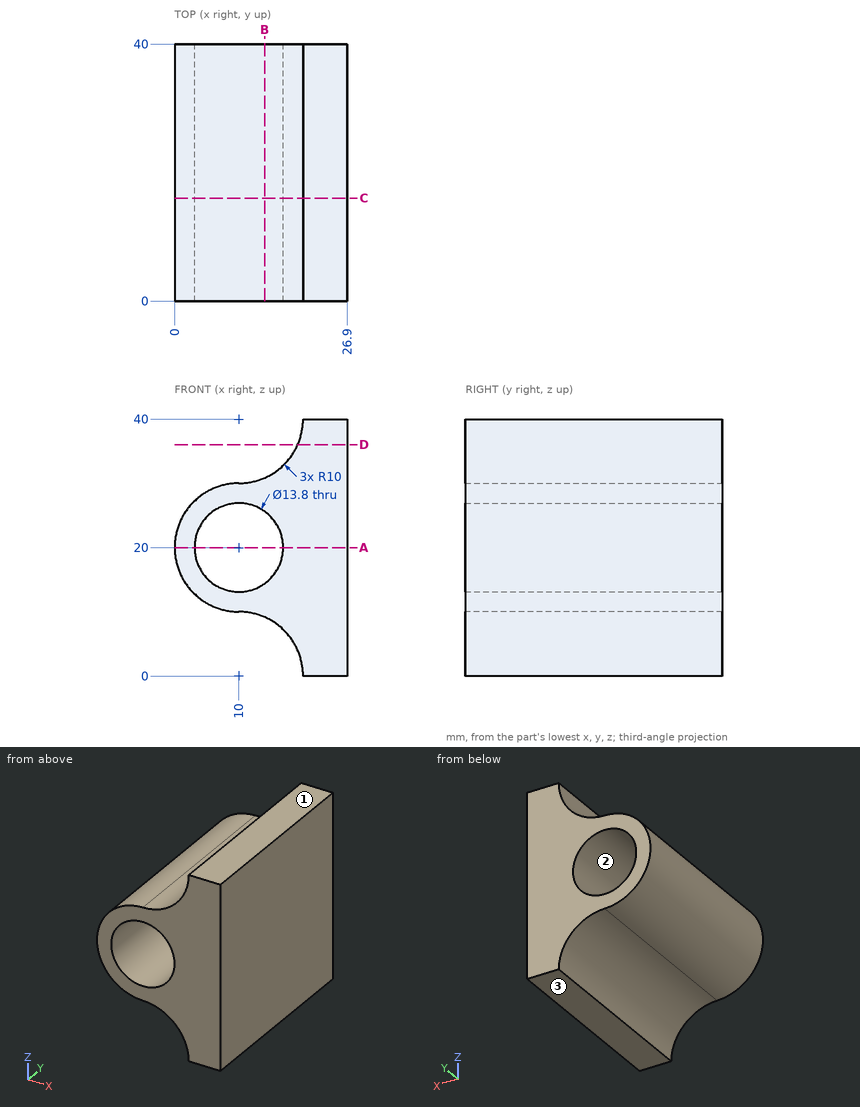
Geometry: see drawing. Coordinates: mm, zero at the bounding-box minimum. Coordinates: 2 decimals unless noted, no trailing zeros. Order: outer loops, then holes, each group sorted by start corner. A loop starts at its lowest first (then second) coordinate and runs counter-clockwise, first axis right, second up. Notation, with made-up numbers: (88, 70.5) - (145, 70.5) arc R15 ccw to (145, 77.5) - close; hole circle Ø11 at (89.5, 6). An arc over 180 degrees is marked (long way). Use one line per item in the form item = value.
1) Section C-C (y = 16). Return loops of the section in (x, z), then the cut area to 3 significant figures.
Solutions:
outline = (10, 10) arc R10 cw to (20, 0) - (26.9, 0) - (26.9, 40) - (20, 40) arc R10 cw to (10, 30) arc R10 ccw to start; hole circle Ø13.8 at (10, 20)
area = 526 mm^2
2) Section A-A (z = 20). Return loops of the section in (x, y).
Solutions:
outline = (0, 0) - (3.1, 0) - (3.1, 40) - (0, 40) - close; (16.9, 0) - (26.9, 0) - (26.9, 40) - (16.9, 40) - close
3) Pin query (flat end, axial travel): pin 1 (11 mm diameter, centred on x = 10, z = 20, fed in from -Y); pin 2 (6 mm diameter, centred on y = 24, z = 10.5, fed in from -X); pin 3 (2 mm diameter, centred on y = 12, z = 22, fed in from -X); pin 4 (10 mm diameter, centred on x = 3, y = 21.5, fed in from +Z). Return the tip coordinate at first contact, or that it passes through.
Solutions:
pin_1 = through
pin_2 = 2.4
pin_3 = 0.05
pin_4 = 29.8
4) Section D-D (z = 36). Return loops of the section in (x, y).
Solutions:
outline = (19.17, 0) - (26.9, 0) - (26.9, 40) - (19.17, 40) - close
5) Mould query, pull axis Z, two halves, no side actions, for the marked faces 1, 2 and 3. Classes: +Z half, -Z half, draft (parallel to the pull), parting line (faces both ways), or undercut.
Solutions:
face_1 = +Z half
face_2 = undercut
face_3 = -Z half
6) Ray query, L1, parallel to Z at x = 10, y = 28.5; L2, parallel to Z at x = 14, y = 30; L3, parallel to X at y = 6, z = 19. Return the intervals inside material, ascending.
Solutions:
L1 = 10 to 13.1, 26.9 to 30
L2 = 9.17 to 14.38, 25.62 to 30.83
L3 = 0.05 to 3.17, 16.83 to 26.9
7) Section B-B (x = 14). Return loops of the section in (y, z), then the cut area to 3 significant figures.
Solutions:
outline = (0, 9.17) - (40, 9.17) - (40, 14.38) - (0, 14.38) - close; (0, 25.62) - (40, 25.62) - (40, 30.83) - (0, 30.83) - close
area = 417 mm^2
